Check sheet for the modelled part. Datum: model origin and axes. Units: mm. A direction names the side the tool comes from. Coordinates: 2 decimals unless noted, no trailing zeros. Order: outer loops, then holes, each group sorted by start corner. A loop starts at its lowest first (then second) coordinate and runs counter-clockwise, first axis right, second up. Notation, with made-up numbers: M -34.75,66.5 L -13.75,66.5 A20 ccw -13.75,80.5 Z; hole C -20.75,21.5 d9. An arc over 180 degrees is marked long. Answer in a Markdown table with one row per item. Add a question column.
from build123d import *

# Parameters (mm, degrees)
SKETCH_1_R          = 7
EXTRUDE_1_DEPTH     = 10
SKETCH_2_R          = 7
EXTRUDE_2_DEPTH     = 5
SKETCH_3_R          = 7
EXTRUDE_3_DEPTH     = 5
SKETCH_4_W          = 1
SKETCH_4_H          = 6.733120112
SKETCH_4_H_2        = 7.353904236
CUT_EXTRUDE_7_DEPTH = 2
SKETCH_5_W          = 27.756401141
SKETCH_5_H          = 22.395981082
CUT_EXTRUDE_8_DEPTH = 10


with BuildPart() as part:
    # Эскиз1 → Вытянуть1 (new body)
    with BuildSketch(Plane(origin=(0, 0, 0), x_dir=(1, 0, 0), z_dir=(0, 1, 0))):
        with Locations(Location((0, 0, 0), (0, 0, 270))):
            Circle(SKETCH_1_R)
        with BuildLine():
            Line((3.85, -1.678541033), (3.85, 1.678541033))
            ThreePointArc((3.85, 1.678541033), (-2.969848481, 2.969848481), (-1.678541033, -3.85))
            Line((-1.678541033, -3.85), (1.678541033, -3.85))
            ThreePointArc((1.678541033, -3.85), (2.969848481, -2.969848481), (3.85, -1.678541033))
        make_face(mode=Mode.SUBTRACT)
    extrude(amount=EXTRUDE_1_DEPTH)

    # Эскиз2 → Вытянуть2 (add)
    with BuildSketch(Plane(origin=(0, 0, 0), x_dir=(1, 0, 0), z_dir=(0, 1, 0))):
        with Locations((12, 0)):
            Circle(SKETCH_2_R)
        with BuildLine():
            Line((15.9, 1.558845727), (15.9, -1.558845727))
            ThreePointArc((15.9, -1.558845727), (14.969848481, -2.969848481), (13.558845727, -3.9))
            Line((13.558845727, -3.9), (10.441154273, -3.9))
            ThreePointArc((10.441154273, -3.9), (9.030151519, 2.969848481), (15.9, 1.558845727))
        make_face(mode=Mode.SUBTRACT)
    extrude(amount=EXTRUDE_2_DEPTH)

    # Эскиз3 → Вытянуть3 (add)
    with BuildSketch(Plane(origin=(0, 0, 0), x_dir=(1, 0, 0), z_dir=(0, 1, 0))):
        with Locations((24, 0)):
            Circle(SKETCH_3_R)
        with BuildLine():
            Line((27.8, 1.846787752), (27.8, -1.846787752))
            ThreePointArc((27.8, -1.846787752), (26.987526151, -2.987526151), (25.846787752, -3.8))
            Line((25.846787752, -3.8), (22.153212248, -3.8))
            ThreePointArc((22.153212248, -3.8), (21.012473849, 2.987526151), (27.8, 1.846787752))
        make_face(mode=Mode.SUBTRACT)
    extrude(amount=EXTRUDE_3_DEPTH)

    # Эскиз4 → Вытянуть7 (cut)
    with BuildSketch(Plane(origin=(0, 10, 0), x_dir=(1, 0, 0), z_dir=(0, 1, 0))):
        with Locations((-0.44096135, 5.658686052)):
            Rectangle(SKETCH_4_W, SKETCH_4_H)
        with Locations((11.258431752, 5.34829399)):
            Rectangle(SKETCH_4_W, SKETCH_4_H_2)
        with Locations((13.407299873, 5.34829399)):
            Rectangle(SKETCH_4_W, SKETCH_4_H_2)
    extrude(amount=-CUT_EXTRUDE_7_DEPTH, mode=Mode.SUBTRACT)

    # Эскиз5 → Вытянуть8 (cut)
    with BuildSketch(Plane(origin=(0, 10, 0), x_dir=(1, 0, 0), z_dir=(0, 1, 0))):
        with Locations((19.658233263, 0.883423561)):
            Rectangle(SKETCH_5_W, SKETCH_5_H)
    extrude(amount=-CUT_EXTRUDE_8_DEPTH, mode=Mode.SUBTRACT)


solid = part.part
1. Section check B-B on y = 6.25. Enter the section's corners in (x, z).
2. Scan lines: line 1 (Z direction, x = 0, y = 3.75); line 2 (X direction, y = 3.5, z = 0); line 3 (Z direction, x = 3.75, y = 1.25). Record each from-to range of solid material in increasing order.
3. Section check A-A on z = 0. Enter the section's corners in (x, y), then the cut area to 3 significant figures.
4. Go/stop test with flat-tipped pins: pin 1 Ø3 at (x, y) = (-2, 6) entering from +Z; pin 2 Ø1.6 at (y, z) = (8.5, -5) entering from -X; pin 3 Ø0.6 at (y, z) = (8.5, -6) entering from +X. Record where each tip stops, or that it passes through.
5. Release check for a two-part mould opening along X. For faces 1 (the flat face through (-3.4, 10, 3)), 2 (the cylindrical face through (-7, 5, 0)), 3 (the flat face through (-0.4, 8, -5.6)), 4 (the flat face through (5.78, 5, 0)) record: released by +X, released by -X, zero draft, split by the parting line, or undercut.
6. Section check C-C on z = 4.25. Enter the section's corners in (x, y), then the cut area to 3 significant figures.
7. Set-up check for faces 5 (the flat face through (0, 5, 3.85)), 6 (the flat face through (-0.941, 9, -5)), 7 (the flat face through (-4, 0, -3)): record each of +Z, -Z, +X, -X, +Y, -Y from which the full face is reachable in a straight line by a thin tool's end or side.
Result sheet:
| question | item | result |
|---|---|---|
| 1 | outline | M 5.78,-3.95 L 5.78,3.95 A7 ccw long Z; hole M -1.68,3.85 A4.2 ccw long 3.85,-1.68 L 3.85,1.68 A4.2 ccw 1.68,3.85 Z |
| 2 | line 1 | -7 to -4.2, 3.85 to 7 |
| 2 | line 2 | -7 to -4.2, 3.85 to 5.78 |
| 2 | line 3 | -5.91 to -1.89, 1.89 to 5.91 |
| 3 | outline | M -7,0 L -4.2,0 L -4.2,10 L -7,10 Z; M 3.85,0 L 5.78,0 L 5.78,10 L 3.85,10 Z |
| 3 | area | 47.3 mm^2 |
| 4 | pin 1 | z = 6.98 |
| 4 | pin 2 | x = -5.6 |
| 4 | pin 3 | x = 4.06 |
| 5 | face 1 | zero draft |
| 5 | face 2 | split by the parting line |
| 5 | face 3 | undercut |
| 5 | face 4 | released by +X |
| 6 | outline | M -5.56,0 L 5.56,0 L 5.56,10 L -5.56,10 Z |
| 6 | area | 111 mm^2 |
| 7 | face 5 | +Y, -Y |
| 7 | face 6 | -Z, +Y |
| 7 | face 7 | +Z, -Z, +X, -X, -Y |
